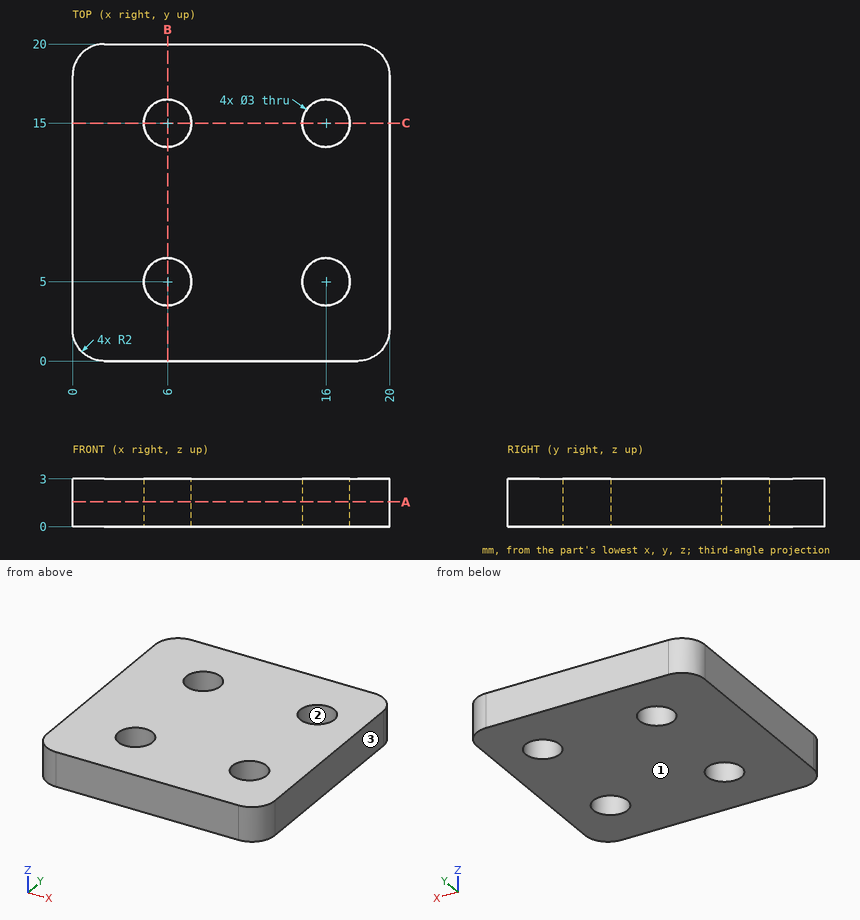
Print and shaded views of the part. All mm, measured from the part's lowest x, y and z. Coordinates: 2 decimals unless noted, no trailing zeros. Order: outer loops, then holes, each group sorted by start corner. A loop starts at its lowest first (then second) coordinate and runs counter-clockwise, first axis right, second up. Notation, with made-up numbers: (-0.75, -12.5) - (41.25, -12.5) arc R21 cw to (41.25, 15.5) - close; hole circle Ø6 at (-30.75, 86). An arc over 180 degrees is marked (long way). Put each result on its own line as item: value.
1. Probe line 1 along Y through (x, z) = (6, 0.7); line 2 along X through (y, z) = (15, 2.3); line 3 along X through (y, z) = (14.25, 2.55). List the from-to ranges inside material, lowest first. Write a range as [from, to].
Answer sheet:
line 1: y = [0, 3.5], [6.5, 13.5], [16.5, 20]
line 2: x = [0, 4.5], [7.5, 14.5], [17.5, 20]
line 3: x = [0, 4.7], [7.3, 14.7], [17.3, 20]
2. Saw through at B-B (x = 6). Write the cut outline in (y, z).
Answer sheet:
outline: (0, 0) - (3.5, 0) - (3.5, 3) - (0, 3) - close; (6.5, 0) - (13.5, 0) - (13.5, 3) - (6.5, 3) - close; (16.5, 0) - (20, 0) - (20, 3) - (16.5, 3) - close
3. Drop a flat-ended pin along its axis: P1, Ø6, axis at x = 8.5, y = 2, coming from the -Z side. Give the stop position or say it passes through.
Answer sheet:
P1: stops at z = 0
4. Saw through at A-A (z = 1.55). Write the cut outline in (x, y), and give its area (3 significant figures).
Answer sheet:
outline: (0, 2) arc R2 ccw to (2, 0) - (18, 0) arc R2 ccw to (20, 2) - (20, 18) arc R2 ccw to (18, 20) - (2, 20) arc R2 ccw to (0, 18) - close; hole circle Ø3 at (6, 5); hole circle Ø3 at (6, 15); hole circle Ø3 at (16, 5); hole circle Ø3 at (16, 15)
area: 368 mm^2
5. Pull direction X, two halves, no side cores. Call the marked faces 1, 2 and 3: pulls with the +X half, pulls with the -X half, needs draft (parallel to the pull), parting line crosses it, or undercut.
Answer sheet:
face 1: needs draft
face 2: undercut
face 3: pulls with the +X half
6. Saw through at C-C (y = 15). Write the cut outline in (x, z).
Answer sheet:
outline: (0, 0) - (4.5, 0) - (4.5, 3) - (0, 3) - close; (7.5, 0) - (14.5, 0) - (14.5, 3) - (7.5, 3) - close; (17.5, 0) - (20, 0) - (20, 3) - (17.5, 3) - close
